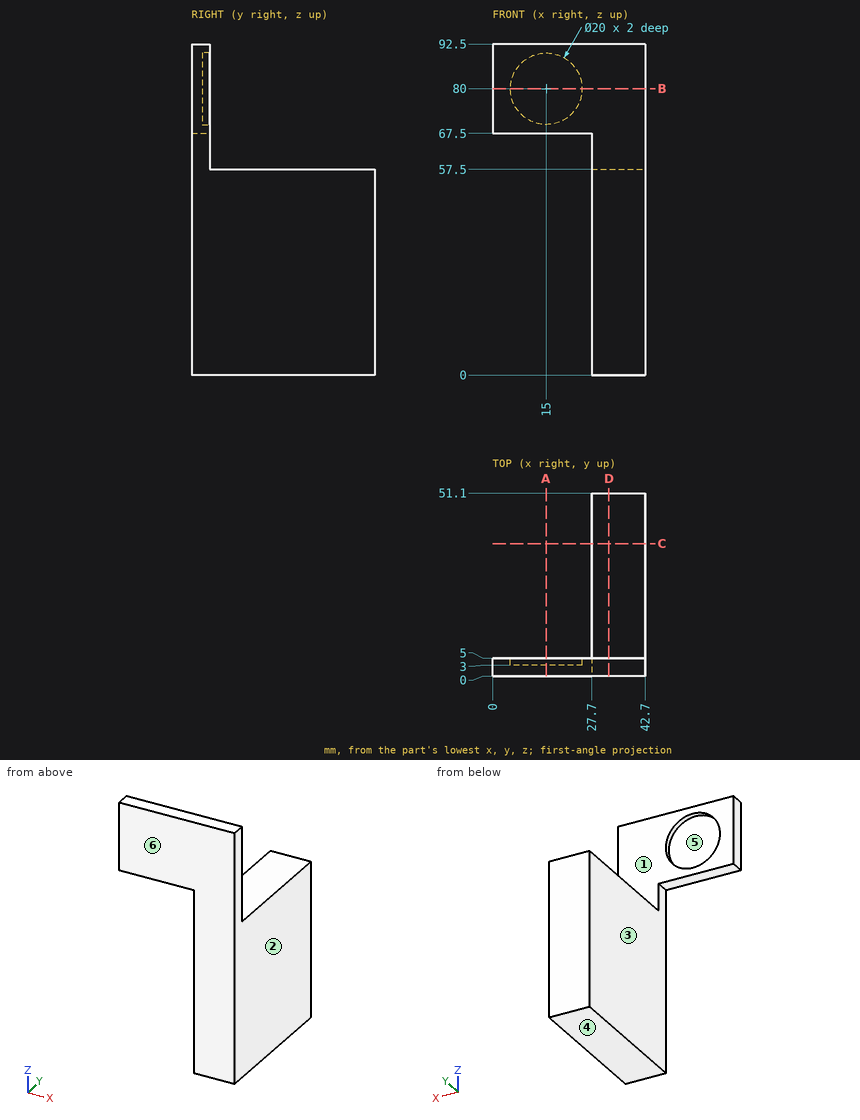
Input: dimensioned drawing with shaded views. Units: mm. Origin: part minimum x, y, z. A direction names the side the tool comes from. Give positions to 0.01 mm unless a question says otherwise; leave off trailing zeros. Loops run counter-clockwise (first coordinate to the right, second up) from the corner with the lowest first, then second, coordinate; pieces in that order, holes last. Notation, with made-up numbers: (-4.75, -1.75) -> (7.25, -1.75) arc R34 ccw to (7.25, 30.25) -> close; hole circle Ø3 at (22, -18). An arc over 180 degrees is marked (long way). Use a Markdown table: item, result. Add a question column.
1) Section query B-B, the plane z = 80. Return the cut outline in (x, y), then the cut area to 4 significant figures.
2) Section query A-A, the plane x = 15. Return the cut outline in (y, z), then the cut area to 3 significant figures.
3) Line query: line 1 along X through (y, z) = (4.45, 80); line 2 along X through (y, z) = (22, 49); line 3 along Z through (x, y) = (34, 48.5). Output: solid intervals per line, ascending. Write a range as [from, to].
4) Reachability of the marked faces 1, 2 and 3 from +Z, -Z, +X, -X, +Y, -Y: full face, straight path, thin tool, end or side. Return the list, or none.
5) Section query D-D, the plane x = 32.5. Return the cut outline in (y, z), then the cut area to 3 significant figures.
6) Section query C-C, the plane y = 37. Return the cut outline in (x, z), then the cut area to 4 significant figures.
7) First-contact query: pin 1 (1.5 mm diameter, centred on x = 12.5, y = 3.5, fed in from -Z); pin 2 (2 mm diameter, centred on x = 25.5, z = 73.5, fed in from +Y); pin 3 (5 mm diameter, centred on x = 32, y = 18, fed in from -Z); pin 4 (12 mm diameter, centred on x = 34.5, y = 39, fed in from +Z). Flat tips, straight axial feed; report the tip coordinate or a pass-through.
8) Pull-direction query (Z, two-part tool) for the marked faces 4, 5 and 6; classes: +Z half, -Z half, draft (parallel to the pull), parting line (faces both ways), or undercut.
Numbers:
| question | item | result |
|---|---|---|
| 1 | outline | (0, 0) -> (42.7, 0) -> (42.7, 5) -> (25, 5) -> (25, 3) -> (5, 3) -> (5, 5) -> (0, 5) -> close |
| 1 | area | 173.5 mm2 |
| 2 | outline | (0, 67.5) -> (5, 67.5) -> (5, 70) -> (3, 70) -> (3, 90) -> (5, 90) -> (5, 92.5) -> (0, 92.5) -> close |
| 2 | area | 85.0 mm2 |
| 3 | line 1 | x = [0, 5], [25, 42.7] |
| 3 | line 2 | x = [27.7, 42.7] |
| 3 | line 3 | z = [0, 57.5] |
| 4 | face 1 | +Z, +X, -X, +Y |
| 4 | face 2 | +Z, -Z, +X, +Y, -Y |
| 4 | face 3 | -Z, -X, +Y, -Y |
| 5 | outline | (0, 0) -> (51.1, 0) -> (51.1, 57.5) -> (5, 57.5) -> (5, 92.5) -> (0, 92.5) -> close |
| 5 | area | 3,110 mm2 |
| 6 | outline | (27.7, 0) -> (42.7, 0) -> (42.7, 57.5) -> (27.7, 57.5) -> close |
| 6 | area | 862.5 mm2 |
| 7 | pin 1 | stops at z = 67.5 |
| 7 | pin 2 | stops at y = 5 |
| 7 | pin 3 | stops at z = 0 |
| 7 | pin 4 | stops at z = 57.5 |
| 8 | face 4 | -Z half |
| 8 | face 5 | undercut |
| 8 | face 6 | draft |
